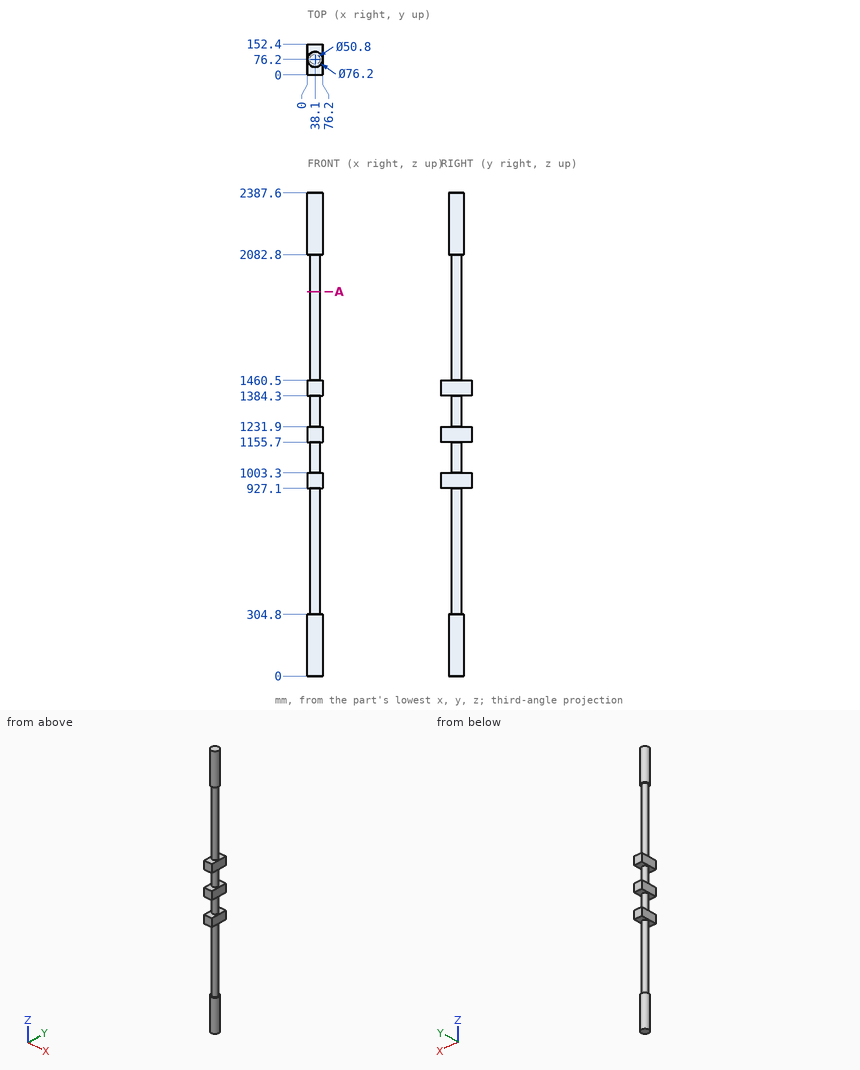
Study the drawing (mm; zero at the part's minimum x, y, z) and answer. Give positions to 0.01 mm unless a question says otherwise; leave off trailing zeros. Order: outer loops, then holes, each group sorted by start corner. A loop starts at its lowest first (then second) coordinate and runs counter-clockwise, first axis right, second up. Notation, with made-up numbers: (-32.5, 39) - (-16.5, 39) arc R25 ccw to (-16.5, 52) - close; hole circle Ø8 at (65, 81). An arc over 180 degrees is marked (long way). Use one line per item in the form item = value. Start each with the question number.
(1) Consider line 1 (Z direction, x = 57, y = 9.5); line 2 (Z direction, x = 13.5, y = 58); line 3 (X direction, y = 79, z = 761). Determine where each line is inside the solid, lowest interval first. Write a range as from..to.
(2) Flat-ended cylindrical pins translate along their axes: pin 1 Ø6 at (y, z) = (55.5, 761.5) entering from -X; pin 2 Ø4 at (x, z) = (46.5, 900.5) entering from -Y; pin 3 Ø10 at (x, y) = (9.5, 17) entering from -Z. Find the tip coordinate at first contact, or state that the pin passes through.
(3) A cutting plane is placed at A-A, the plane z = 1899.5. Write down the section's boundary in (x, y).
Ans:
q1.line_1 = 927.1..1003.3, 1155.7..1231.9, 1384.3..1460.5
q1.line_2 = 0..304.8, 927.1..1003.3, 1155.7..1231.9, 1384.3..1460.5, 2082.8..2387.6
q1.line_3 = 12.85..63.35
q2.pin_1 = 19.88
q2.pin_2 = 51.62
q2.pin_3 = 927.1
q3.outline = circle Ø50.8 at (38.1, 76.2)
